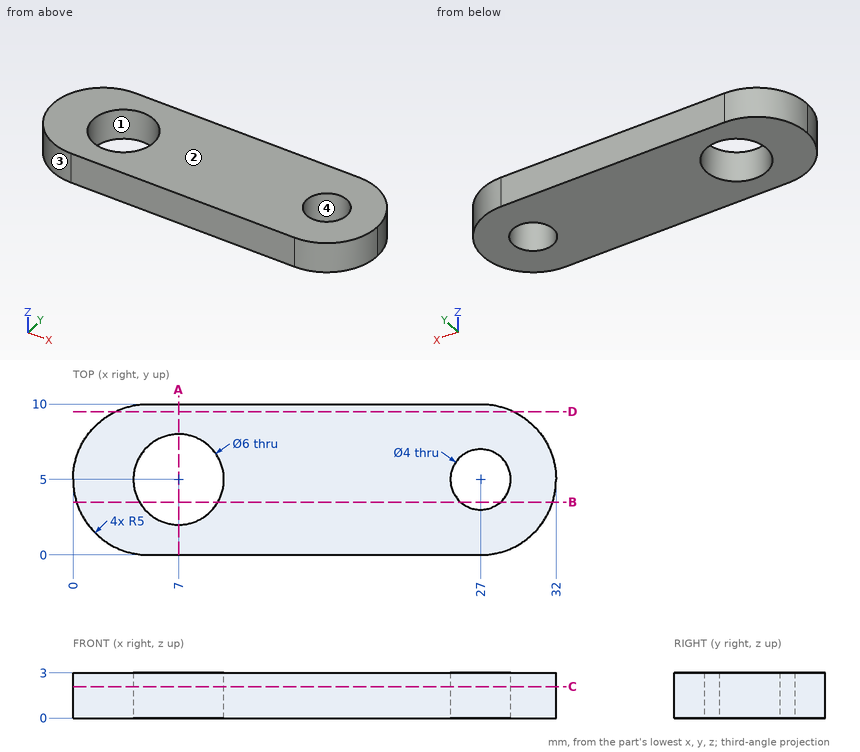
Check sheet for the drawn part. Datum: minimum x, y, z corner. Units: mm. Round coordinates to 2 decimals unless told otherwise and drop trailing zeros. Loops run counter-clockwise (first coordinate to the right, second up) from the corner with the lowest first, then second, coordinate; pieces in that order, holes last. Notation, with made-up numbers: (-29, 76) - (10, 76) arc R26 ccw to (10, 99) - close; hole circle Ø8 at (54, 76.25). An arc over 180 degrees is marked (long way). Answer as a JSON object with one key per item and string values. Group by question number.
Q1. Sectioned sample at D-D, the plane y = 9.5. Enter the section's corners in (x, z), plus the area to 3 significant figures.
Q2. Sectioned sample at C-C, the plane z = 2.1. Count the separate pieces of the cut face and the enclosed holes in it, plus the area to 3 significant figures.
Q3. Gauge pin test, flat end, axial feed: P1, Ø1.5, axis at y = 6.5, z = 1.5, coming from the +X side. Record the tip position at first contact, or that the pin passes through.
Q4. Sectioned sample at B-B, the plane y = 3.5. Enter the section's corners in (x, z).
Q5. Mould release check, pull along Y, two halves, no side actions. Record for the marked faces 1, 2, 3 and 4: released by +Y, released by -Y, zero draft, split by the parting line, or undercut.
Q6. Scan lines: line 1 along Y through (x, z) = (7, 0.65); line 2 along Y through (x, z) = (27, 1.3); line 3 along X through (y, z) = (6, 2.15). Record each from-to range of solid material in increasing order. Write a range as [from, to].
Q7. Sectioned sample at A-A, the plane x = 7. Enter the section's corners in (y, z), plus the area to 3 significant figures.
Solution:
{
 "1": {"outline": "(2.82, 0) - (29.18, 0) - (29.18, 3) - (2.82, 3) - close", "area": "79.1 mm²"},
 "2": {"separate pieces": "1", "enclosed holes": "2", "area": "258 mm²"},
 "3": {"P1": "stops at x = 31.94"},
 "4": {"outline": "(0.23, 0) - (4.4, 0) - (4.4, 3) - (0.23, 3) - close; (9.6, 0) - (25.68, 0) - (25.68, 3) - (9.6, 3) - close; (28.32, 0) - (31.77, 0) - (31.77, 3) - (28.32, 3) - close"},
 "5": {"face 1": "undercut", "face 2": "zero draft", "face 3": "released by -Y", "face 4": "undercut"},
 "6": {"line 1": "y = [0, 2], [8, 10]", "line 2": "y = [0, 3], [7, 10]", "line 3": "x = [0.1, 4.17], [9.83, 25.27], [28.73, 31.9]"},
 "7": {"outline": "(0, 0) - (2, 0) - (2, 3) - (0, 3) - close; (8, 0) - (10, 0) - (10, 3) - (8, 3) - close", "area": "12.0 mm²"}
}
